Geometry check sheet. Reference: the model listing, model coordinates, mm. Face numbers are marked on the shaded views. Give positions to 0.01 mm unless a question says otherwise; leave off trailing zeros. Write each loop counter-clockwise with the first axis right and the second up, starting at its lowest first coordinate (ties: lowest second). Pieces come first, ordered by that corner, then holes. Notation, with made-up numbers: (35, 79.5) - (62, 79.5) arc R20 ccw to (62, 90.5) - close; hole circle Ø6 at (-36.5, 89). An arc over 180 degrees is marked (long way). Write item = value, one per line. Start each with the question number.
(1) Section check C-C, the plane z = 3. Enter the section's corners in (x, y), plus the area to 3 significant figures.
(2) Depth check by flat-ended pin: pin 1 Ø1.5 at (x, y) = (0, 6.5) entering from +Z; pin 2 Ø12 at (x, y) = (5.5, -4) entering from -Z. Enter the tip coordinate at first touch or a pass-through.
(3) Section check A-A, the plane x = 0. Enter the section's corners in (y, z), plus the area to 4 significant figures.
(4) Section check D-D, the plane z = 0.8. Enter the section's corners in (x, y).
(5) Thickness scan on L1, parallel to Y at x = 0, z = 3.7; L2, parallel to Z at x = 0.5, y = -5.5; L3, parallel to Y at x = 0, z = 1.9. Record the ranges inside material, lowest first.
(6) Draft check along Y on the marked faces 1, 2 and 3. Enter one of: pulls with the +Y half, pulls with the -Y half, needs draft (parallel to the pull), parting line crosses it, or undercut.
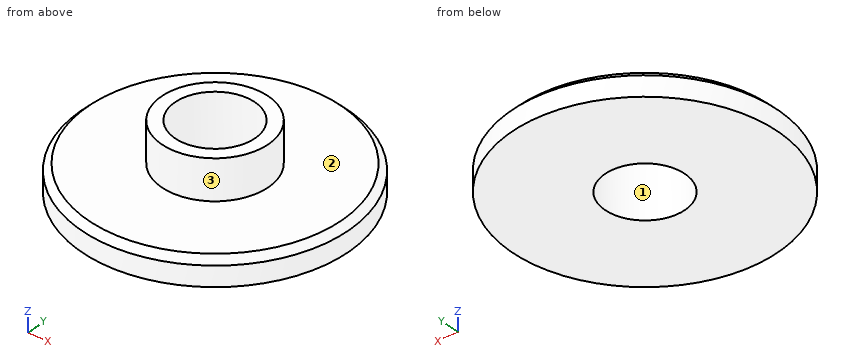
Autodesk Inventor part; units mm, degrees
ref_plane "YZ Plane" through (0, 0, 0) normal (1, 0, 0) x (0, 1, 0)
ref_plane "XZ Plane" through (0, 0, 0) normal (0, 1, 0) x (-1, 0, 0)
ref_plane "XY Plane" through (0, 0, 0) normal (0, 0, 1) x (1, 0, 0)
sketch "Sketch1" plane through (0, 0, 0) normal (0, 0, 1) x (1, 0, 0)
  circle A0 centre (0, 0) radius 10
  circle A1 centre (0, 0) radius 3
  dimension "d0" = 20
  dimension "d1" = 6
extrude "Extrusion1" add sketch "Sketch1" along normal blind 2
sketch "Sketch2" plane through (0, 0, 2) normal (0, 0, 1) x (1, 0, 0)
  circle A0 centre (0, 0) radius 4
  circle A1 centre (0, 0) radius 3
  dimension "d4" = 8
extrude "Extrusion2" add sketch "Sketch2" along normal blind 3
chamfer "Chamfer1" distance 0.5 angle 45 1 edges at (-10, 0, 2)
properties part number "end eff servo-conector"
Model answer:
q1.outline = circle Ø8 at (0, 0); hole circle Ø6 at (0, 0)
q1.area = 22.0 mm²
q2.pin_1 = 2
q2.pin_2 = 0
q3.outline = (-10, 0) - (-3, 0) - (-3, 5) - (-4, 5) - (-4, 2) - (-9.5, 2) - (-10, 1.5) - close; (3, 0) - (10, 0) - (10, 1.5) - (9.5, 2) - (4, 2) - (4, 5) - (3, 5) - close
q3.area = 33.75 mm²
q4.outline = circle Ø20 at (0, 0); hole circle Ø6 at (0, 0)
q5.L1 = -4 to -3, 3 to 4
q5.L2 = 0 to 2
q5.L3 = -9.6 to -3, 3 to 9.6
q6.face_1 = undercut
q6.face_2 = needs draft
q6.face_3 = parting line crosses it
